The listing builds one solid part. Answer for the finished solid, in the listing's coordinates (mm). A direction names the side the tool comes from. Give positions to 0.01 mm unless a question says otherwise; leave off trailing zeros. Write each loop counter-clockwise with the first axis right and the second up, starting at its lowest first coordinate (ties: lowest second). Pieces come first, ordered by that corner, then holes. Notation, with made-up numbers: (3, -19) - (37, -19) arc R13 ccw to (37, -5) - close; hole circle Ø9 at (33.25, -26). An arc over 180 degrees is marked (long way). Answer as CSV lines item,"result". Start each with the question number.
(1) For a pull along Y with two mould halves and no side action, classify faces 1 (the face through (-30.5, 4, 22)), 2 (the face through (0, 16, 26)), 3 (the face through (0.497, 13.585, 21.486)), 4 (the face through (39.036, -0.986, -0.668)) as pulls with the +Y half, pulls with the -Y half, needs draft (parallel to the pull), parting line crosses it, or undercut.
(2) Find section C-C (z = -14.5). Write down the section's boundary in (x, y), then the cut area to 3 significant figures.
(3) Straight lines are drawn through the part: probe 1 along Z at (x, y) = (20, 10.75); probe 2 along Y at (x, z) = (32, 2.5); probe 3 along Y at (x, z) = (-4.5, 9). For each, find the intervals that lie inside material, in ascending order.
(4) For faces 5 (the face through (32, 1, -5.343)), 6 (the face through (0, 7, -25.5)), 7 (the face through (-42, 0, 5.667)), 8 (the face through (30.5, 1, 0)), 9 (the face through (-33.03, 0.86, 18.91)), determine the directions among +Z, -Z, +X, -X, +Y, -Y from which every point of the face is accessible in a straight line to the end or side of a thin tool.
(5) Each of these flat-tipped pins is pushed along its axis until it touches: pin 1 Ø24.5 at (x, z) = (9, 1.5) entering from +Y; pin 2 Ø2.5 at (x, z) = (-32, -11.5) entering from +Y; pin 3 Ø0.6 at (x, y) = (41, -1) entering from -Z; pin 4 Ø5.5 at (y, z) = (4, 15.5) entering from +X. Where does it stop, or does it pass through?
(6) Find section D-D (x = 33.5). Write down the section's boundary in (y, z).
(7) Find section A-A (x = -42.5). Write down the section's boundary in (y, z), then the cut area to 3 significant figures.
(8) Find section B-B (y = 11). Write down the section's boundary in (x, z), then the cut area to 3 significant figures.
from build123d import *

# Parameters (mm, degrees)
SKETCH1_W           = 71
SKETCH1_H           = 61
SKETCH1_W_2         = 61
SKETCH1_H_2         = 51
BOSS_EXTRUDE1_DEPTH = 16
SKETCH2_W           = 71
SKETCH2_H           = 61
BOSS_EXTRUDE2_DEPTH = 2
SKETCH3_W           = 11.849749017
SKETCH3_H           = 16
CUT_EXTRUDE1_DEPTH  = 12
FILLET1_R           = 3
SKETCH4_W           = 15
SKETCH4_H           = 16
CUT_EXTRUDE2_DEPTH  = 12
SKETCH5_W           = 21
SKETCH5_H           = 8
CUT_EXTRUDE3_DEPTH  = 12
SKETCH6_W           = 51
SKETCH6_H           = 8
CUT_EXTRUDE4_DEPTH  = 12
CHAMFER1_SIZE       = 1
SKETCH8_W           = 21
SKETCH8_H           = 8
CUT_EXTRUDE5_DEPTH  = 14
SKETCH9_W           = 71
SKETCH9_H           = 3
BOSS_EXTRUDE4_DEPTH = 5
CHAMFER3_SIZE       = 2
CHAMFER3_SIZE2      = 1.154700538
SKETCH10_W          = 71
SKETCH10_H          = 3
BOSS_EXTRUDE5_DEPTH = 5
CHAMFER4_SIZE       = 2
CHAMFER4_SIZE2      = 1.154700538
SKETCH11_W          = 5
SKETCH11_H          = 10
BOSS_EXTRUDE6_DEPTH = 2
CHAMFER5_SIZE       = 2
CHAMFER5_SIZE2      = 3.464101615
SKETCH12_W          = 14
SKETCH12_H          = 5
BOSS_EXTRUDE7_DEPTH = 14
CHAMFER6_SIZE       = 2
SKETCH13_R          = 2
CUT_EXTRUDE6_DEPTH  = 14
FILLET2_R           = 3
SKETCH14_W          = 10
SKETCH14_H          = 2
BOSS_EXTRUDE8_DEPTH = 10
SKETCH15_R          = 1.5
CUT_EXTRUDE7_DEPTH  = 10
CHAMFER7_SIZE       = 3
CHAMFER8_SIZE       = 3
FILLET3_R           = 3


with BuildPart() as part:
    # Sketch1 → Boss-Extrude1 (new body)
    with BuildSketch(Plane(origin=(0, 0, 0), x_dir=(1, 0, 0), z_dir=(0, 1, 0))):
        Rectangle(SKETCH1_W, SKETCH1_H)
        Rectangle(SKETCH1_W_2, SKETCH1_H_2, mode=Mode.SUBTRACT)
    extrude(amount=BOSS_EXTRUDE1_DEPTH)

    # Sketch2 → Boss-Extrude2 (add)
    with BuildSketch(Plane.XZ):
        Rectangle(SKETCH2_W, SKETCH2_H)
    extrude(amount=BOSS_EXTRUDE2_DEPTH)

    # Sketch3 → Cut-Extrude1 (cut)
    with BuildSketch(Plane(origin=(-30.5, 0, 0), x_dir=(0, 0, -1), z_dir=(1, 0, 0))):
        with Locations((-13.884589143, 8)):
            Rectangle(SKETCH3_W, SKETCH3_H)
    extrude(amount=-CUT_EXTRUDE1_DEPTH, mode=Mode.SUBTRACT)

    # Fillet1
    fillet1_edges = [part.edges().sort_by_distance(p)[0] for p in [
        (-33, 0, 19.809463651),
        (-33, 0, 7.959714634),
    ]]
    fillet(fillet1_edges, radius=FILLET1_R)

    # Sketch4 → Cut-Extrude2 (cut)
    with BuildSketch(Plane.ZY.offset(-30.5)):
        with Locations((-18, 8)):
            Rectangle(SKETCH4_W, SKETCH4_H)
        with Locations((18, 8)):
            Rectangle(SKETCH4_W, SKETCH4_H)
    extrude(amount=-CUT_EXTRUDE2_DEPTH, mode=Mode.SUBTRACT)

    # Sketch5 → Cut-Extrude3 (cut)
    with BuildSketch(Plane.ZY.offset(-30.5)):
        with Locations((0, 12)):
            Rectangle(SKETCH5_W, SKETCH5_H)
    extrude(amount=-CUT_EXTRUDE3_DEPTH, mode=Mode.SUBTRACT)

    # Sketch6 → Cut-Extrude4 (cut)
    with BuildSketch(Plane(origin=(-30.5, 0, 0), x_dir=(0, 0, -1), z_dir=(1, 0, 0))):
        with Locations((0, 12)):
            Rectangle(SKETCH6_W, SKETCH6_H)
    extrude(amount=-CUT_EXTRUDE4_DEPTH, mode=Mode.SUBTRACT)

    # Chamfer1
    chamfer1_edges = [part.edges().sort_by_distance(p)[0] for p in [
        (2.5, 0, -25.5),
        (2.5, 0, 25.5),
    ]]
    chamfer(chamfer1_edges, length=CHAMFER1_SIZE)

    # Sketch8 → Cut-Extrude5 (cut)
    with BuildSketch(Plane.ZY.offset(-30.5)):
        with Locations((0, 4)):
            Rectangle(SKETCH8_W, SKETCH8_H)
    extrude(amount=-CUT_EXTRUDE5_DEPTH, mode=Mode.SUBTRACT)

    # Sketch9 → Boss-Extrude4 (add)
    with BuildSketch(Plane.XY.offset(-25.5)):
        with Locations((0, 14.5)):
            Rectangle(SKETCH9_W, SKETCH9_H)
    extrude(amount=BOSS_EXTRUDE4_DEPTH)

    # Chamfer3
    chamfer3_edges = [part.edges().sort_by_distance(p)[0] for p in [
        (0, 13, -20.5),
    ]]
    chamfer3_side = [part.faces().sort_by_distance(p)[0] for p in [
        (0, 13, -23),
    ]]
    chamfer(chamfer3_edges, length=CHAMFER3_SIZE, length2=CHAMFER3_SIZE2, reference=chamfer3_side[0])

    # Sketch10 → Boss-Extrude5 (add)
    with BuildSketch(Plane(origin=(0, 0, 25.5), x_dir=(-1, 0, 0), z_dir=(0, 0, -1))):
        with Locations((0, 14.5)):
            Rectangle(SKETCH10_W, SKETCH10_H)
    extrude(amount=BOSS_EXTRUDE5_DEPTH)

    # Chamfer4
    chamfer4_edges = [part.edges().sort_by_distance(p)[0] for p in [
        (0, 13, 20.5),
    ]]
    chamfer4_side = [part.faces().sort_by_distance(p)[0] for p in [
        (0, 13, 23),
    ]]
    chamfer(chamfer4_edges, length=CHAMFER4_SIZE, length2=CHAMFER4_SIZE2, reference=chamfer4_side[0])

    # Sketch11 → Boss-Extrude6 (add)
    with BuildSketch(Plane(origin=(0, 0, 0), x_dir=(1, 0, 0), z_dir=(0, 1, 0))):
        with Locations((33, 0.342687242)):
            Rectangle(SKETCH11_W, SKETCH11_H)
    extrude(amount=BOSS_EXTRUDE6_DEPTH)

    # Chamfer5
    chamfer5_edges = [part.edges().sort_by_distance(p)[0] for p in [
        (35.5, 2, -0.342687242),
    ]]
    chamfer5_side = [part.faces().sort_by_distance(p)[0] for p in [
        (35.5, 15.077350269, 21.136003145),
    ]]
    chamfer(chamfer5_edges, length=CHAMFER5_SIZE, length2=CHAMFER5_SIZE2, reference=chamfer5_side[0])

    # Sketch12 → Boss-Extrude7 (add)
    with BuildSketch(Plane.ZY.offset(35.5)):
        with Locations((-1.332725664, 0.5)):
            Rectangle(SKETCH12_W, SKETCH12_H)
    extrude(amount=BOSS_EXTRUDE7_DEPTH)

    # Chamfer6
    chamfer6_edges = [part.edges().sort_by_distance(p)[0] for p in [
        (-35.5, 3, -1.332725664),
    ]]
    chamfer(chamfer6_edges, length=CHAMFER6_SIZE)

    # Sketch13 → Cut-Extrude6 (cut)
    with BuildSketch(Plane(origin=(0, 3, 0), x_dir=(1, 0, 0), z_dir=(0, 1, 0))):
        with Locations(Location((-42.5, 1.332725664, 0), (0, 0, 270))):
            Circle(SKETCH13_R)
    extrude(amount=-CUT_EXTRUDE6_DEPTH, mode=Mode.SUBTRACT)

    # Fillet2
    fillet2_edges = [part.edges().sort_by_distance(p)[0] for p in [
        (-49.5, 0.5, -8.332725664),
        (-49.5, 0.5, 5.667274336),
    ]]
    fillet(fillet2_edges, radius=FILLET2_R)

    # Sketch14 → Boss-Extrude8 (add)
    with BuildSketch(Plane(origin=(35.5, 0, 0), x_dir=(0, 0, -1), z_dir=(1, 0, 0))):
        with Locations((0.342687242, -1)):
            Rectangle(SKETCH14_W, SKETCH14_H)
    extrude(amount=BOSS_EXTRUDE8_DEPTH)

    # Sketch15 → Cut-Extrude7 (cut)
    with BuildSketch(Plane(origin=(0, 0, 0), x_dir=(1, 0, 0), z_dir=(0, 1, 0))):
        with Locations(Location((40.5, 0.342687242, 0), (0, 0, 270))):
            Circle(SKETCH15_R)
    extrude(amount=-CUT_EXTRUDE7_DEPTH, mode=Mode.SUBTRACT)

    # Chamfer7
    chamfer7_edges = [part.edges().sort_by_distance(p)[0] for p in [
        (45.5, -1, 4.657312758),
        (45.5, -1, -5.342687242),
    ]]
    chamfer(chamfer7_edges, length=CHAMFER7_SIZE)

    # Chamfer8
    # the kernel refuses this chamfer: 3 mm, written as the material it adds along each edge
    with BuildSketch(Plane(origin=(35.5, -2, 4.657312758), x_dir=(0.9996219169112968, 0, -0.02749587661058648), z_dir=(0, 1, 0)), Plane(origin=(35.5, 0, -5.342687242), x_dir=(0.9996219169112968, 0, 0.02749587661058648), z_dir=(0, -1, 0))) as chamfer8_piece_1:
        Polygon((CHAMFER8_SIZE * 0.999621916911, -CHAMFER8_SIZE * 0.0274958766106), (-CHAMFER8_SIZE * 0.0274958766106, -CHAMFER8_SIZE * 0.999621916911), (0, 0), align=None)
    extrude(amount=2)

    # Fillet3
    # the kernel refuses this fillet: 3 mm, written as the material it adds along each edge
    with BuildSketch(Plane(origin=(-35.5, 12.5, 5.667274336), x_dir=(0, 0, 1), z_dir=(0, -1, 0))) as fillet3_piece_1_section:
        with BuildLine():
            CenterArc((FILLET3_R, FILLET3_R), FILLET3_R, 180, 90)
            Line((0, FILLET3_R), (0, 0))
            Line((0, 0), (FILLET3_R, 0))
        make_face()
    fillet3_piece_1 = extrude(amount=14.5, mode=Mode.PRIVATE)
    fillet3_piece_1 = split(fillet3_piece_1, bisect_by=Plane(origin=(-37.935900015, 2.564099985, 5.657679593), z_dir=(-0.7071067811865477, 0.7071067811865475, 0)), keep=Keep.TOP, mode=Mode.PRIVATE)
    fillet3_piece_1 = split(fillet3_piece_1, bisect_by=Plane(origin=(-38.08120002, 3, 5.657679593), z_dir=(0, -1, 0)), keep=Keep.TOP, mode=Mode.PRIVATE)
    add(fillet3_piece_1)
    with BuildSketch(Plane(origin=(-35.5, 12.5, 5.667274336), x_dir=(0, 0, 1), z_dir=(0, -1, 0))) as fillet3_piece_2_section:
        with BuildLine():
            CenterArc((FILLET3_R, FILLET3_R), FILLET3_R, 180, 90)
            Line((0, FILLET3_R), (0, 0))
            Line((0, 0), (FILLET3_R, 0))
        make_face()
    fillet3_piece_2 = extrude(amount=14.5, mode=Mode.PRIVATE)
    fillet3_piece_2 = split(fillet3_piece_2, bisect_by=Plane(origin=(-36.308682262, 4.191317738, 6.44717053), z_dir=(0.7071067811865477, -0.7071067811865475, 0)), keep=Keep.TOP, mode=Mode.PRIVATE)
    fillet3_piece_2 = split(fillet3_piece_2, bisect_by=Plane(origin=(-35.911576349, 3.794211825, 7.959714634), z_dir=(0, 0, -1)), keep=Keep.TOP, mode=Mode.PRIVATE)
    fillet3_piece_2 = split(fillet3_piece_2, bisect_by=Plane(origin=(-35.911576349, 3, 6.44717053), z_dir=(0, 1, 0)), keep=Keep.TOP, mode=Mode.PRIVATE)
    add(fillet3_piece_2)
    with BuildSketch(Plane(origin=(-35.5, 12.5, 5.667274336), x_dir=(0, 0, 1), z_dir=(0, -1, 0))) as fillet3_piece_3_section:
        with BuildLine():
            CenterArc((FILLET3_R, FILLET3_R), FILLET3_R, 180, 90)
            Line((0, FILLET3_R), (0, 0))
            Line((0, 0), (FILLET3_R, 0))
        make_face()
    fillet3_piece_3 = extrude(amount=14.5, mode=Mode.PRIVATE)
    fillet3_piece_3 = split(fillet3_piece_3, bisect_by=Plane(origin=(-38.099888212, 2.400111788, 6.295666552), z_dir=(0.7071067811865477, -0.7071067811865475, 0)), keep=Keep.TOP, mode=Mode.PRIVATE)
    fillet3_piece_3 = split(fillet3_piece_3, bisect_by=Plane(origin=(-36.191024286, 0.491247862, 7.959714634), z_dir=(0, 0, -1)), keep=Keep.TOP, mode=Mode.PRIVATE)
    fillet3_piece_3 = split(fillet3_piece_3, bisect_by=Plane(origin=(-36.191024286, 3, 6.295666552), z_dir=(0, -1, 0)), keep=Keep.TOP, mode=Mode.PRIVATE)
    add(fillet3_piece_3)
    with BuildSketch(Plane(origin=(-35.5, 12.5, 5.667274336), x_dir=(0, 0, 1), z_dir=(0, -1, 0))) as fillet3_piece_4_section:
        with BuildLine():
            CenterArc((FILLET3_R, FILLET3_R), FILLET3_R, 180, 90)
            Line((0, FILLET3_R), (0, 0))
            Line((0, 0), (FILLET3_R, 0))
        make_face()
    fillet3_piece_4 = extrude(amount=14.5, mode=Mode.PRIVATE)
    fillet3_piece_4 = split(fillet3_piece_4, bisect_by=Plane(origin=(-35.48926289, -0.06844391, 7.959714634), z_dir=(0, 0, 1)), keep=Keep.TOP, mode=Mode.PRIVATE)
    fillet3_piece_4 = fillet3_piece_4 - Plane(origin=(-35.48926289, 3, 10.959714634), x_dir=(0, -1, 0), z_dir=(-1, 0, 0)) * Cylinder(3, 41, mode=Mode.PRIVATE)
    fillet3_piece_4 = split(fillet3_piece_4, bisect_by=Plane(origin=(-35.48926289, 3, 8.232443119), z_dir=(0, -1, 0)), keep=Keep.TOP, mode=Mode.PRIVATE)
    add(fillet3_piece_4)
    with BuildSketch(Plane(origin=(-35.5, -2, -8.332725664), x_dir=(0, 0, -1), z_dir=(0, 1, 0))) as fillet3_piece_5_section:
        with BuildLine():
            CenterArc((FILLET3_R, FILLET3_R), FILLET3_R, 180, 90)
            Line((0, FILLET3_R), (0, 0))
            Line((0, 0), (FILLET3_R, 0))
        make_face()
    fillet3_piece_5 = extrude(amount=14.5, mode=Mode.PRIVATE)
    fillet3_piece_5 = split(fillet3_piece_5, bisect_by=Plane(origin=(-38.090184906, 2.409815094, -9.014565132), z_dir=(0.7071067811865477, -0.7071067811865475, 0)), keep=Keep.TOP, mode=Mode.PRIVATE)
    fillet3_piece_5 = split(fillet3_piece_5, bisect_by=Plane(origin=(-36.171856175, 3, -9.014565132), z_dir=(0, -1, 0)), keep=Keep.TOP, mode=Mode.PRIVATE)
    add(fillet3_piece_5)
    with BuildSketch(Plane(origin=(-35.5, -2, -8.332725664), x_dir=(0, 0, -1), z_dir=(0, 1, 0))) as fillet3_piece_6_section:
        with BuildLine():
            CenterArc((FILLET3_R, FILLET3_R), FILLET3_R, 180, 90)
            Line((0, FILLET3_R), (0, 0))
            Line((0, 0), (FILLET3_R, 0))
        make_face()
    fillet3_piece_6 = extrude(amount=14.5, mode=Mode.PRIVATE)
    fillet3_piece_6 = split(fillet3_piece_6, bisect_by=Plane(origin=(-37.935900015, 2.564099985, -8.32313092), z_dir=(-0.7071067811865477, 0.7071067811865475, 0)), keep=Keep.TOP, mode=Mode.PRIVATE)
    fillet3_piece_6 = split(fillet3_piece_6, bisect_by=Plane(origin=(-38.08120002, 3, -8.32313092), z_dir=(0, -1, 0)), keep=Keep.TOP, mode=Mode.PRIVATE)
    add(fillet3_piece_6)
    with BuildSketch(Plane(origin=(-35.5, -2, -8.332725664), x_dir=(0, 0, -1), z_dir=(0, 1, 0))) as fillet3_piece_7_section:
        with BuildLine():
            CenterArc((FILLET3_R, FILLET3_R), FILLET3_R, 180, 90)
            Line((0, FILLET3_R), (0, 0))
            Line((0, 0), (FILLET3_R, 0))
        make_face()
    fillet3_piece_7 = extrude(amount=14.5, mode=Mode.PRIVATE)
    fillet3_piece_7 = split(fillet3_piece_7, bisect_by=Plane(origin=(-36.295704825, 4.204295175, -9.186455327), z_dir=(0.7071067811865477, -0.7071067811865475, 0)), keep=Keep.TOP, mode=Mode.PRIVATE)
    fillet3_piece_7 = split(fillet3_piece_7, bisect_by=Plane(origin=(-35.8942731, 3, -9.186455327), z_dir=(0, 1, 0)), keep=Keep.TOP, mode=Mode.PRIVATE)
    add(fillet3_piece_7)


solid = part.part
Result set:
1,face 1,"undercut"
1,face 2,"pulls with the +Y half"
1,face 3,"undercut"
1,face 4,"needs draft"
2,outline,"(-35.5, -2) - (35.5, -2) - (35.5, 0) - (-30.5, 0) - (-30.5, 8) - (-35.5, 8) - close"
2,area,"182 mm^2"
3,probe 1,"-30.5 to -25.5, 25.5 to 30.5"
3,probe 2,"-2 to 2"
3,probe 3,"-2 to 0"
4,face 5,"+X, +Y"
4,face 6,"+X"
4,face 7,"+Z, -X, +Y, -Y"
4,face 8,"+Y"
4,face 9,"+X, -X, +Y"
5,pin 1,"y = 0"
5,pin 2,"y = 8"
5,pin 3,"z = -5.34"
5,pin 4,"through"
6,outline,"(-2, -30.5) - (16, -30.5) - (16, -20.5) - (14.15, -20.5) - (13, -22.5) - (13, -25.5) - (1, -25.5) - (0, -24.5) - (0, -5.34) - (1.15, -5.34) - (1.15, 4.66) - (0, 4.66) - (0, 24.5) - (1, 25.5) - (13, 25.5) - (13, 22.5) - (14.15, 20.5) - (16, 20.5) - (16, 30.5) - (-2, 30.5) - close"
7,outline,"(-2, -8.33) - (3, -8.33) - (3, -3.33) - (-2, -3.33) - close; (-2, 0.67) - (3, 0.67) - (3, 5.67) - (-2, 5.67) - close"
7,area,"50.0 mm^2"
8,outline,"(-35.5, -30.5) - (35.5, -30.5) - (35.5, -25.5) - (-35.5, -25.5) - close; (-35.5, 25.5) - (35.5, 25.5) - (35.5, 30.5) - (-35.5, 30.5) - close"
8,area,"710 mm^2"
